The model under review builds one solid part; all positions refer to its coordinate system, in mm. A direction names the side the tool comes from. Give positions to 0.01 mm unless a question says otherwise; leave off trailing zeros. Order: outer loops, then holes, each group sorted by start corner. A loop starts at its lowest first (then second) coordinate and runs counter-clockwise, first axis right, second up. Notation, with made-up numbers: (81.25, 86) - (86.25, 86) arc R23 cw to (86.25, 108) - close; hole circle Ø9 at (5.5, 25.25). An arc over 180 degrees is marked (long way). Use CSV: the item, a comma, the result in double quotes. Start each with the question number.
1. To check wall thickness, follow line 1 (Z direction, x = 0.2, y = 30); line 2 (Y direction, x = 0.4, z = -20); line 3 (Z direction, x = 2.75, y = 27.5). State the ranges of each line that lie inside material, in increasing order. Write a range as [from, to].
2. Take a section at D-D, the plane y = 42.5. State the section outline as (x, z) points, then the cut area to 3 significant figures.
3. Draft analysis for pull direction Z (two halves, no side actions). For faces 3 (the cylindrical face through (0.43, 11.96, -23.32)), 4 (the cylindrical face through (8.34, 61.05, 48.66)), state which applies: released by +Z, released by -Z, zero draft, split by the parting line, or undercut.
4. Take a section at B-B, the plane z = -20. State the section outline as (x, y) points.
5. Take a section at C-C, the plane z = -47.5. Count the separate pieces of the cut face and the enclosed holes in it, then the cut area to 3 significant figures.
6. For pin 1 (2.5 mm diameter, centred on x = 2.5, z = -19.5, fed in from +Y); pin 2 (10.5 mm diameter, centred on y = 30, z = 45, fed in from +X); pin 3 (1.5 mm diameter, centred on y = 14, z = -29, fed in from +X), all flat-tipped, find the tip position at first contact; note any pin that passes through.
7. Take a section at A-A, the plane y = 30. State the section outline as (x, z) points, then the cut area to 3 significant figures.
8. Machinability: for faces 1 (the conical face through (1.11, 28.57, -40.46)), 2 (the flat face through (2.7, 57, -37)), which of the approach directions +Z, -Z, +X, -X, +Y, -Y give a long, thin tool a straight path to every point of the face, cutting with its end or side? Answer none if there is none.
```python
from build123d import *

# Parameters (mm, degrees)
SKETCH15_W                                     = 5
SKETCH15_H                                     = 60
EXTRUDE_THIN2_DEPTH                            = 60
SKETCH16_R                                     = 5
SKETCH17_R                                     = 3.5
CUT_EXTRUDE4_DEPTH                             = 137.839321834
CSK_FOR_M8_FLAT_HEAD_MACHINE_SCREW4_AT_2_COUNT = 2
CSK_FOR_M8_FLAT_HEAD_MACHINE_SCREW4_AT_2_PITCH = 29.154759474
SKETCH37_W                                     = 26
SKETCH37_H                                     = 11
F_2CUTS_DEPTH                                  = 89.600225733
F_2CUTS_DEPTH_BACK                             = 89.600225733


with BuildPart() as part:
    # Sketch15 → Extrude-Thin2 (new, symmetric)
    with BuildSketch(Plane.XY):
        with Locations((2.5, 30)):
            Rectangle(SKETCH15_W, SKETCH15_H)
    extrude(amount=EXTRUDE_THIN2_DEPTH, both=True)

    # Sweep2: sweep along a curve in space
    with BuildLine() as sweep2_path:
        Line((5, 60, 60), (5, 60, -60))
    # Sketch16 → Sweep2 (sweep)
    with BuildSketch(Plane(origin=(0, 0, -60), x_dir=(-1, 0, 0), z_dir=(0, 0, -1))):
        with Locations((-5, 60)):
            Circle(SKETCH16_R)
    sweep(path=sweep2_path.line)

    # Sketch17 → Cut-Extrude4 (cut, through all)
    with BuildSketch(Plane.XY.offset(60)):
        with Locations((5, 60)):
            Circle(SKETCH17_R)
    extrude(amount=-CUT_EXTRUDE4_DEPTH, mode=Mode.SUBTRACT)

    # Sketch18 → CSK for M8 Flat Head Machine Screw4 (revolve, cut)
    with BuildSketch(Plane(origin=(5, 30, 45), x_dir=(0, 0, -1), z_dir=(0, 1, 0))):
        Polygon((0, 0), (0, 5), (4.5, 5), (4.5, 4.15), (8.65, 0), align=None)
    csk_for_m8_flat_head_machine_screw4 = revolve(axis=Axis((11.35, 30, 45), (-1, 0, 0)), mode=Mode.SUBTRACT)

    # CSK for M8 Flat Head Machine Screw4 at 2: CSK for M8 Flat Head Machine Screw4 ×2
    with Locations(*[Vector(0, -0.5144957554275265, -0.8574929257125442) * (i * CSK_FOR_M8_FLAT_HEAD_MACHINE_SCREW4_AT_2_PITCH) for i in range(1, CSK_FOR_M8_FLAT_HEAD_MACHINE_SCREW4_AT_2_COUNT)]):
        add(csk_for_m8_flat_head_machine_screw4, mode=Mode.SUBTRACT)

    # Mirror7: CSK for M8 Flat Head Machine Screw4 across plane
    add(csk_for_m8_flat_head_machine_screw4.mirror(Plane.XY), mode=Mode.SUBTRACT)

    # Mirror7 copy 1 sketch → Mirror7 copy 1 (revolve, cut)
    with BuildSketch(Plane(origin=(5, 15, -20), x_dir=(0, 0, 1), z_dir=(0, 1, 0))):
        Polygon((0, 0), (0, -5), (4.5, -5), (4.5, -4.15), (8.65, 0), align=None)
    revolve(axis=Axis((11.35, 15, -20), (1, 0, 0)), mode=Mode.SUBTRACT)

    # Sketch37 → 2Cuts (cut, two sides)
    with BuildSketch(Plane(origin=(5, 0, 0), x_dir=(0, 0, -1), z_dir=(1, 0, 0))) as f_2cuts_sk:
        with Locations((24, 59.5)):
            Rectangle(SKETCH37_W, SKETCH37_H)
        with Locations((-24, 59.5)):
            Rectangle(SKETCH37_W, SKETCH37_H)
    extrude(amount=F_2CUTS_DEPTH, mode=Mode.SUBTRACT)
    extrude(f_2cuts_sk.sketch, amount=-F_2CUTS_DEPTH_BACK, mode=Mode.SUBTRACT)


solid = part.part
```
Determined:
1,line 1,"z = [-60, -49.5], [-40.5, 40.5], [49.5, 60]"
1,line 2,"y = [0, 10.5], [19.5, 54]"
1,line 3,"z = [-60, -50.89], [-39.11, 39.11], [50.89, 60]"
2,outline,"(0, -60) - (5, -60) - (5, 60) - (0, 60) - close"
2,area,"600 mm²"
3,face 3,"undercut"
3,face 4,"zero draft"
4,outline,"(0, 0) - (5, 0) - (5, 6.35) - (0.85, 10.5) - (0, 10.5) - close; (0, 19.5) - (0.85, 19.5) - (5, 23.65) - (5, 54) - (0, 54) - close"
5,separate pieces,"2"
5,enclosed holes,"1"
5,area,"264 mm²"
6,pin 1,"stops at y = 54"
6,pin 2,"stops at x = 1.6"
6,pin 3,"stops at x = 5"
7,outline,"(0, -60) - (5, -60) - (5, -53.65) - (0.85, -49.5) - (0, -49.5) - close; (0, -40.5) - (0.85, -40.5) - (5, -36.35) - (5, 36.35) - (0.85, 40.5) - (0, 40.5) - close; (0, 49.5) - (0.85, 49.5) - (5, 53.65) - (5, 60) - (0, 60) - close"
7,area,"476 mm²"
8,face 1,"+X"
8,face 2,"+X, -X, +Y"
